```python
from build123d import *

# Parameters (mm, degrees)
SKETCH1_R           = 1.575
SKETCH1_R_2         = 2.5
BOSS_EXTRUDE1_DEPTH = 5
SKETCH3_W           = 13.4
SKETCH3_H           = 5
BOSS_EXTRUDE2_DEPTH = 5


with BuildPart() as part:
    # Sketch1 → Boss-Extrude1 (new body)
    with BuildSketch(Plane.XY):
        with BuildLine():
            Line((-139.300035894, 89.802561211), (-24.748737342, -24.748737342))
            ThreePointArc((-24.748737342, -24.748737342), (24.748737342, -24.748737342), (24.748737342, 24.748737342))
            Line((24.748737342, 24.748737342), (-54.672802234, 104.170276917))
            Line((-54.672802234, 104.170276917), (-76.622366364, 126.119841047))
            ThreePointArc((-76.622366364, 126.119841047), (-78.790093877, 129.364074535), (-79.551298552, 133.190908859))
            Line((-79.551298552, 133.190908859), (-79.551298552, 164.551298552))
            Line((-79.551298552, 164.551298552), (-89.351298552, 164.551298552))
            Line((-89.351298552, 164.551298552), (-89.351298552, 169.551298552))
            Line((-89.351298552, 169.551298552), (-96.351298552, 169.551298552))
            Line((-96.351298552, 169.551298552), (-96.351298552, 174.551298552))
            Line((-96.351298552, 174.551298552), (-109.751298552, 174.551298552))
            Line((-109.751298552, 174.551298552), (-109.751298552, 169.551298552))
            Line((-109.751298552, 169.551298552), (-109.751298552, 164.551298552))
            Line((-109.751298552, 164.551298552), (-102.201298552, 164.551298552))
            Line((-102.201298552, 164.551298552), (-102.201298552, 159.701298552))
            Line((-102.201298552, 159.701298552), (-126.901298552, 159.701298552))
            Line((-126.901298552, 159.701298552), (-126.901298552, 164.551298552))
            Line((-126.901298552, 164.551298552), (-119.351298552, 164.551298552))
            Line((-119.351298552, 164.551298552), (-119.351298552, 169.551298552))
            Line((-119.351298552, 169.551298552), (-119.351298552, 174.551298552))
            Line((-119.351298552, 174.551298552), (-132.751298552, 174.551298552))
            Line((-132.751298552, 174.551298552), (-132.751298552, 169.551298552))
            Line((-132.751298552, 169.551298552), (-139.751298552, 169.551298552))
            Line((-139.751298552, 169.551298552), (-139.751298552, 164.551298552))
            Line((-139.751298552, 164.551298552), (-149.551298552, 164.551298552))
            Line((-149.551298552, 164.551298552), (-149.551298552, 114.551298552))
            ThreePointArc((-149.551298552, 114.551298552), (-146.88708219, 101.157378419), (-139.300035894, 89.802561211))
        make_face()
        with Locations((-20.506096654, -20.506096654)):
            Circle(SKETCH1_R, mode=Mode.SUBTRACT)
        with Locations((-12.727922061, -12.727922061)):
            Circle(SKETCH1_R_2, mode=Mode.SUBTRACT)
        with Locations((-56.568542495, 14.142135624)):
            Circle(SKETCH1_R, mode=Mode.SUBTRACT)
        with BuildLine():
            ThreePointArc((-45.891723759, 8.555498392), (-45.891723759, 12.670859859), (-41.776362292, 12.670859859))
            Line((-41.776362292, 12.670859859), (-32.583974137, 3.478471704))
            ThreePointArc((-32.583974137, 3.478471704), (-32.583974137, -0.636889763), (-36.699335604, -0.636889763))
            Line((-36.699335604, -0.636889763), (-45.891723759, 8.555498392))
        make_face(mode=Mode.SUBTRACT)
        with Locations((20.506096654, -20.506096654)):
            Circle(SKETCH1_R, mode=Mode.SUBTRACT)
        with Locations((12.727922061, 12.727922061)):
            Circle(SKETCH1_R_2, mode=Mode.SUBTRACT)
        with Locations((-20.506096654, 20.506096654)):
            Circle(SKETCH1_R, mode=Mode.SUBTRACT)
        with BuildLine():
            ThreePointArc((-35.001785669, 56.922095886), (-35.001785669, 60.457629791), (-31.466251763, 60.457629791))
            Line((-31.466251763, 60.457629791), (-10.253048327, 39.244426356))
            ThreePointArc((-10.253048327, 39.244426356), (-10.253048327, 35.70889245), (-13.788582233, 35.70889245))
            Line((-13.788582233, 35.70889245), (-35.001785669, 56.922095886))
        make_face(mode=Mode.SUBTRACT)
        with Locations((-14.142135624, 56.568542495)):
            Circle(SKETCH1_R, mode=Mode.SUBTRACT)
        with Locations((20.506096654, 20.506096654)):
            Circle(SKETCH1_R, mode=Mode.SUBTRACT)
        with Locations((-114.551298552, 84.551298552)):
            Circle(SKETCH1_R, mode=Mode.SUBTRACT)
        with BuildLine():
            ThreePointArc((-101.4698231, 123.390133317), (-101.4698231, 126.925667223), (-97.934289194, 126.925667223))
            Line((-97.934289194, 126.925667223), (-76.721085759, 105.712463787))
            ThreePointArc((-76.721085759, 105.712463787), (-76.721085759, 102.176929881), (-80.256619665, 102.176929881))
            Line((-80.256619665, 102.176929881), (-101.4698231, 123.390133317))
        make_face(mode=Mode.SUBTRACT)
        with Locations((-64.396887007, 105.308740477)):
            Circle(SKETCH1_R, mode=Mode.SUBTRACT)
        with Locations((-136.551298552, 152.551298552)):
            Circle(SKETCH1_R, mode=Mode.SUBTRACT)
        with Locations((-92.551298552, 152.551298552)):
            Circle(SKETCH1_R, mode=Mode.SUBTRACT)
        with BuildLine():
            ThreePointArc((-68.235804384, 90.156114601), (-68.235804384, 93.691648507), (-64.700270479, 93.691648507))
            Line((-64.700270479, 93.691648507), (-43.487067043, 72.478445072))
            ThreePointArc((-43.487067043, 72.478445072), (-43.487067043, 68.942911166), (-47.022600949, 68.942911166))
            Line((-47.022600949, 68.942911166), (-68.235804384, 90.156114601))
        make_face(mode=Mode.SUBTRACT)
    extrude(amount=-BOSS_EXTRUDE1_DEPTH)

    # Sketch3 → Boss-Extrude2 (add)
    with BuildSketch(Plane.XY):
        with Locations((-126.051298552, 177.051298552)):
            Rectangle(SKETCH3_W, SKETCH3_H)
        with Locations((-103.051298552, 177.051298552)):
            Rectangle(SKETCH3_W, SKETCH3_H)
    extrude(amount=-BOSS_EXTRUDE2_DEPTH)


solid = part.part
```
Verification items for the finished model (mm, model axes). A direction names the side the tool comes from. Coordinates: 2 decimals unless noted, no trailing zeros. Write each loop counter-clockwise with the first axis right and the second up, starting at its lowest first coordinate (ties: lowest second). Pieces come first, ordered by that corner, then holes. Notation, with made-up numbers: (1, 37) - (9, 37) arc R30 cw to (9, 70) - close; hole circle Ø4 at (-21.75, 1). An arc over 180 degrees is marked (long way). Write item = value, one per line.
Q1. Access from +Z, -Z, +X, -X, +Y, -Y to the whole of each face (thin tool, end or side, straight path). Record for faces 4 (the face through (-89.351, 167, -2)), 5 (the face through (-119.351, 172, -2)), 6 (the face through (-41.231, 3.895, -2.465)).
Answer:
face_4 = +Z, -Z, +X, +Y
face_5 = +Z, -Z, +Y
face_6 = +Z, -Z
Q2. Cross-section at B-B (z = -2.05). Give the number of separate pieces and of enclosed holes in the cut face, plus the area to 3 significant figures.
Answer:
separate_pieces = 1
enclosed_holes = 16
area = 16,400 mm²
Q3. Cross-section at C-C (x = 0). Enter the section's corners in (y, z), plus the area to 3 significant figures.
Answer:
outline = (-35, -5) - (49.5, -5) - (49.5, 0) - (-35, 0) - close
area = 422 mm²
Q4. Cross-section at A-A (y = 48.5). Enter the section's corners in (x, z).
Answer:
outline = (-98, -5) - (-26.58, -5) - (-26.58, 0) - (-98, 0) - close; (-19.51, -5) - (1, -5) - (1, 0) - (-19.51, 0) - close
Q5. Material ranges on L1, parallel to Y at x = 19.5, z = -2; L2, parallel to X at y = 163, z = -1.1; L3, parallel to Y at x = 20, z = -0.9, recorded low to high. Write a range as from..to.
Answer:
L1 = -29.06..-21.72, -19.29..19.29, 21.72..30
L2 = -149.55..-126.9, -102.2..-79.55
L3 = -28.72..-22, -19.01..19.01, 22..29.5
Q6. Go/stop test with flat-tipped pins: pin 1 Ø4.5 at (x, y) = (-12.73, -12.73) entering from +Z; pin 2 Ø1 at (x, z) = (-44, -3.5) entering from -Y; pin 3 Ø1 at (x, z) = (-77, -4.5) entering from +Y; pin 4 Ø2.5 at (y, z) = (167.5, -3) entering from +X. Record where each tip stops, or that it passes through.
Answer:
pin_1 = through
pin_2 = -6
pin_3 = 127.12
pin_4 = -89.35
Q7. Mould release check, pull along Y, two halves, no side actions. Record for faces 1 (the face through (-145, 164.551, -2)), 2 (the face through (-149.551, 140, -2)), 3 (the face through (15.112, 13.479, -2.465)): released by +Y, released by -Y, zero draft, split by the parting line, or undercut.
Answer:
face_1 = released by +Y
face_2 = zero draft
face_3 = undercut
